from build123d import *

# Parameters (mm, degrees)
F0_W     = 52.5
F0_H     = 15
F1_DEPTH = 10
F2_R     = 2.5
F3_DEPTH = 25
F4_W     = 15
F4_H     = 10
F5_DEPTH = 60
F6_R     = 2.5
F7_DEPTH = 5


with BuildPart() as f1:
    # F0 (on Top) → F1 (new body)
    with BuildSketch(Plane.XY):
        with Locations((-36.5180644393, 6.5659499308)):
            Rectangle(F0_W, F0_H)
    extrude(amount=F1_DEPTH)

    # F2 (on face) → F3 (cut)
    with BuildSketch(Plane.XY.offset(10)):
        with Locations((-15.2680644393, 6.5659499308)):
            Circle(F2_R)
        with Locations((-57.7680644393, 6.5659499308)):
            Circle(F2_R)
    extrude(amount=-F3_DEPTH, mode=Mode.SUBTRACT)

    # F4 (on face) → F5 (join)
    with BuildSketch(Plane(origin=(-62.7680644393, 0, 0), x_dir=(0, -1, 0), z_dir=(-1, 0, 0))):
        with Locations((-6.5659499308, 5)):
            Rectangle(F4_W, F4_H)
    extrude(amount=F5_DEPTH)

    # F6 (on face) → F7 (join)
    with BuildSketch(Plane(origin=(0, 0, 0), x_dir=(1, 0, 0), z_dir=(0, 0, -1))):
        with Locations((-117.7680644393, -6.5659499308)):
            Circle(F6_R)
    extrude(amount=F7_DEPTH)

    # F10 (on offset) → F11 (revolve)
    with BuildSketch(Plane(origin=(-117.7680644393, 0, 0), x_dir=(0, -1, 0), z_dir=(-1, 0, 0))):
        with BuildLine():
            Line((-6.5659499308, -5), (-9.0659499308, -5))
            ThreePointArc((-9.0659499308, -5), (-8.3337168838, -6.767766953), (-6.5659499308, -7.5))
            Line((-6.5659499308, -7.5), (-6.5659499308, -5))
        make_face()
    revolve(axis=Axis((-117.7680644393, 6.5659499308, -6.25), (0, 0, -1)))


solid = f1.part
Could you check a few things on this model? Use its own coordinates, in mm. Give positions to 0.01 mm unless a question says otherwise; leave off trailing zeros. Loops run counter-clockwise (first coordinate to the right, second up) from the corner with the lowest first, then second, coordinate; pieces in that order, holes last. Notation, with made-up numbers: (59.5, -8) -> (91.5, -8) arc R9 ccw to (91.5, 0) -> close; hole circle Ø5 at (39, 85.5). An arc over 180 degrees is marked (long way). Answer as CSV lines item,"result". Start each with the question number.
(1) We'd pull the mould along X, two halves only. Please class faces 1 (the flat face through (-66, -0.934, 5)), 2 (the cylindrical face through (-115.38, 5.82, -2.46)), 3 (the cylindrical face through (-60.266, 6.676, 5.07)): released by +X, released by -X, zero draft, split by the parting line, or undercut.
(2) I need wall thicknesses on probe 1 along X at (y, z) = (5, 7); probe 2 along Z at (x, y) = (-28, 6); probe 3 along Y at (x, z) = (-58, 4.5). Which ranges of each line are inside material? Lowest first, please.
(3) I'm going to push a flat-ended pin straight in: pin 1 Ø8 at (x, y) = (-57.77, 6.57) entering from -Z. Where does the tip first touch, or does it pass through?
(4) If we section it at C-C on x = -88: Write out the boundary of the cut face in (y, z), then the cut area to 3 significant figures.
(5) If we section it at A-A on y = 5.5: Write out the boundary of the cut face in (x, z).
(6) If we section it at D-D on z = -6: Write out the boundary of the cut face in (x, y), then the cut area to 3 significant figures.
(7) If we section it at B-B on z = 8: Write out the boundary of the cut face in (x, y).
Computed:
1,face 1,"zero draft"
1,face 2,"split by the parting line"
1,face 3,"undercut"
2,probe 1,"x = -122.77 to -59.72, -55.82 to -17.22, -13.32 to -10.27"
2,probe 2,"z = 0 to 10"
2,probe 3,"y = -0.93 to 4.08, 9.06 to 14.07"
3,pin 1,"stops at z = 0"
4,outline,"(-0.93, 0) -> (14.07, 0) -> (14.07, 10) -> (-0.93, 10) -> close"
4,area,"150 mm2"
5,outline,"(-122.77, 0) -> (-120.03, 0) -> (-120.03, -5) arc R2.26 ccw to (-115.51, -5) -> (-115.51, 0) -> (-60.03, 0) -> (-60.03, 10) -> (-122.77, 10) -> close; (-55.51, 0) -> (-17.53, 0) -> (-17.53, 10) -> (-55.51, 10) -> close; (-13.01, 0) -> (-10.27, 0) -> (-10.27, 10) -> (-13.01, 10) -> close"
6,outline,"circle Ø4.58 at (-117.77, 6.57)"
6,area,"16.5 mm2"
7,outline,"(-122.77, -0.93) -> (-10.27, -0.93) -> (-10.27, 14.07) -> (-122.77, 14.07) -> close; hole circle Ø5 at (-57.77, 6.57); hole circle Ø5 at (-15.27, 6.57)"
